Source: CAD feature listing. Evaluate the final solid. Frame: model axes, mm. Face numbers are marked on the shaded views. A direction names the side the tool comes from. Give positions to 0.01 mm unless a question says otherwise; leave off trailing zeros. Write each loop counter-clockwise with the first axis right and the second up, starting at its lowest first coordinate (ties: lowest second). Pieces come first, ordered by that corner, then holes. Notation, with made-up numbers: (-1, 1.25) - (34, 1.25) arc R10 cw to (34, 17.25) - close; hole circle Ø3 at (-30.5, 80.5). An arc over 180 degrees is marked (long way). Answer as a JSON object with one key per item and string values. Group by question number.
from build123d import *

# Parameters (mm, degrees)
F0_W     = 126.65081
F0_H     = 28.956786
F0_R     = 4.613754
F1_DEPTH = 12
F2_R     = 1
F3_R     = 1
F4_R     = 1


with BuildPart() as f1:
    # F0 (on Top) → F1 (new body)
    with BuildSketch(Plane.XY):
        Rectangle(F0_W, F0_H)
        with Locations((-38.348339, 0)):
            Circle(F0_R, mode=Mode.SUBTRACT)
        with BuildLine():
            ThreePointArc((0, -5.238965), (-5.238965, 0), (0, 5.238965))
            Line((0, 5.238965), (37.103504, 5.238965))
            ThreePointArc((37.103504, 5.238965), (42.342469, 0), (37.103504, -5.238965))
            Line((37.103504, -5.238965), (0, -5.238965))
        make_face(mode=Mode.SUBTRACT)
    extrude(amount=F1_DEPTH)

    # F2
    f2_edges = [f1.edges().sort_by_distance(p)[0] for p in [
        (-42.962094, 0, 12),
        (42.342469, 0, 12),
    ]]
    fillet(f2_edges, radius=F2_R)

    # F3
    f3_edges = [f1.edges().sort_by_distance(p)[0] for p in [
        (0, -14.478393, 0),
        (0, 14.478393, 0),
        (63.325405, 0, 0),
        (-63.325405, 0, 0),
    ]]
    fillet(f3_edges, radius=F3_R)

    # F4
    f4_edges = [f1.edges().sort_by_distance(p)[0] for p in [
        (0, -14.478393, 12),
        (63.325405, 0, 12),
        (0, 14.478393, 12),
        (-63.325405, 0, 12),
    ]]
    fillet(f4_edges, radius=F4_R)


solid = f1.part
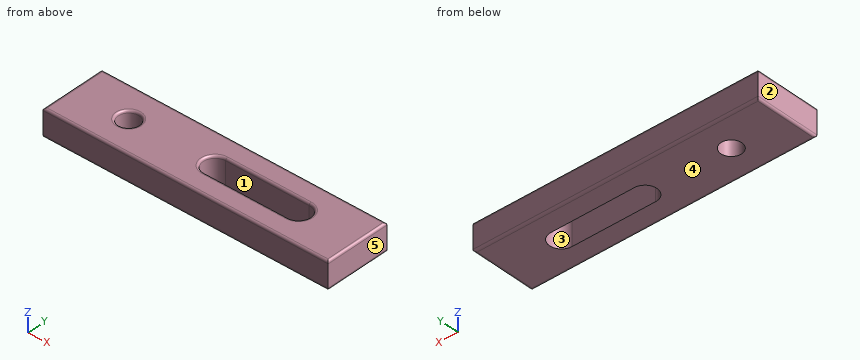
Q1. Reachability of the marked faces 1 and 2 from +Z, -Z, +X, -X, +Y, -Y: full face, straight path, thin tool, end or side. Return the list, or none.
Q2. Ray query, probe 1 along X at (y, z) = (-2.5, 5.75); probe 2 along X at (y, z) = (-1.25, 2.5); probe 3 along Y at (x, z) = (26, 8). Return the intervals inside material, ascending. Write a range as [from, to].
Q3. Draft query along X for the marked faces 3, 4 and 5. Return one class per face: released by +X, released by -X, zero draft, split by the parting line, or undercut.
Q4. Section A-A on x = 32. Return the cut outline in (y, z).
Q5. Section C-C on z = 8. Return the cut outline in (x, y), then the cut area to 3 significant figures.
Q6. Section B-B on y = 0. Return the cut outline in (x, z).
Taken from the geometry:
{
 "1": {"face 1": "+Z, -Z", "face 2": "+Z, -Z, -X, +Y, -Y"},
 "2": {"probe 1": "x = [-63.33, -42.23], [-34.47, -4.6], [41.71, 63.33]", "probe 2": "x = [-63.33, -42.79], [-33.91, -5.09], [42.19, 63.33]", "probe 3": "y = [-14.48, -5.24], [5.24, 14.48]"},
 "3": {"face 3": "undercut", "face 4": "zero draft", "face 5": "released by +X"},
 "4": {"outline": "(-14.48, 1) arc R1 ccw to (-13.48, 0) - (-5.24, 0) - (-5.24, 11) arc R1 ccw to (-6.24, 12) - (-13.48, 12) arc R1 ccw to (-14.48, 11) - close; (5.24, 0) - (13.48, 0) arc R1 ccw to (14.48, 1) - (14.48, 11) arc R1 ccw to (13.48, 12) - (6.24, 12) arc R1 ccw to (5.24, 11) - close"},
 "5": {"outline": "(-63.33, -14.48) - (63.33, -14.48) - (63.33, 14.48) - (-63.33, 14.48) - close; hole circle Ø9.23 at (-38.35, 0); hole (0, -5.24) - (37.1, -5.24) arc R5.24 ccw to (37.1, 5.24) - (0, 5.24) arc R5.24 ccw to start", "area": "3,130 mm²"},
 "6": {"outline": "(-63.33, 1) arc R1 ccw to (-62.33, 0) - (-42.96, 0) - (-42.96, 11) arc R1 ccw to (-43.96, 12) - (-62.33, 12) arc R1 ccw to (-63.33, 11) - close; (-33.73, 0) - (-5.24, 0) - (-5.24, 11) arc R1 ccw to (-6.24, 12) - (-32.73, 12) arc R1 ccw to (-33.73, 11) - close; (42.34, 0) - (62.33, 0) arc R1 ccw to (63.33, 1) - (63.33, 11) arc R1 ccw to (62.33, 12) - (43.34, 12) arc R1 ccw to (42.34, 11) - close"}
}
